Geometry check sheet. Reference: the model listing, model coordinates, mm. Face numbers are marked on the shaded views. A direction names the side the tool comes from. Coordinates: 2 decimals unless noted, no trailing zeros. Write each loop counter-clockwise with the first axis right and the second up, starting at its lowest first coordinate (ties: lowest second). Pieces come first, ordered by that corner, then holes. Notation, with made-up numbers: M 52.5,88 L 75.5,88 A23 ccw 75.5,114 Z; hole C 58.25,21.5 d10. An arc over 180 degrees is marked long. Write each question's results on one line, items separated by ' | '.
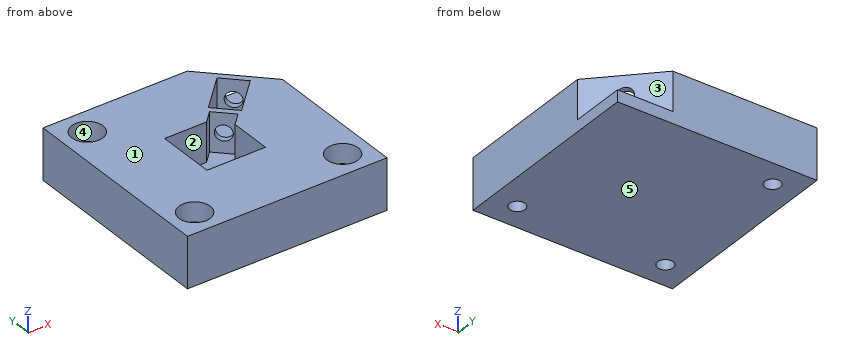
```python
from build123d import *

# Parameters (mm, degrees)
F0_W      = 51.2
F0_H      = 51.2
F0_R      = 2
F1_DEPTH  = 3
F2_R      = 2
F3_DEPTH  = 5
F4_R      = 4
F5_DEPTH  = 5
F6_R      = 2
F7_DEPTH  = 2
F8_R      = 3.5
F9_DEPTH  = 11
F10_R     = 2
F11_DEPTH = 4
F13_DEPTH = 9


with BuildPart() as f1:
    # F0 (on Top) → F1 (new body)
    with BuildSketch(Plane.XY):
        Rectangle(F0_W, F0_H)
        with Locations((-19, -19)):
            Circle(F0_R, mode=Mode.SUBTRACT)
        with Locations((19, -19)):
            Circle(F0_R, mode=Mode.SUBTRACT)
        with Locations((-19, 19)):
            Circle(F0_R, mode=Mode.SUBTRACT)
    extrude(amount=F1_DEPTH)

    # F2 (on face) → F3 (join)
    with BuildSketch(Plane.XY.offset(3)):
        Polygon((11.4, 25.6), (-25.6, 25.6), (-25.6, -25.6), (25.6, -25.6), (25.6, 11.4), align=None)
        with Locations((-19, -19)):
            Circle(F2_R, mode=Mode.SUBTRACT)
        with Locations((19, -19)):
            Circle(F2_R, mode=Mode.SUBTRACT)
        with Locations((-19, 19)):
            Circle(F2_R, mode=Mode.SUBTRACT)
        Polygon((-7.5, -7.5), (-7.5, 7.5), (3.2573593129, 7.5), (6.0857864376, 10.3284271247), (10.3284271247, 6.0857864376), (7.5, 3.2573593129), (7.5, -7.5), align=None, mode=Mode.SUBTRACT)
    extrude(amount=F3_DEPTH)

    # F4 (on face) → F5 (join)
    with BuildSketch(Plane.XY.offset(8)):
        Polygon((11.4, 25.6), (-25.6, 25.6), (-25.6, -25.6), (25.6, -25.6), (25.6, 11.4), align=None)
        with Locations((-19, -19)):
            Circle(F4_R, mode=Mode.SUBTRACT)
        with Locations((19, -19)):
            Circle(F4_R, mode=Mode.SUBTRACT)
        with Locations((-19, 19)):
            Circle(F4_R, mode=Mode.SUBTRACT)
        Polygon((-7.5, -7.5), (-7.5, 7.5), (3.2573593129, 7.5), (6.0857864376, 10.3284271247), (10.3284271247, 6.0857864376), (7.5, 3.2573593129), (7.5, -7.5), align=None, mode=Mode.SUBTRACT)
    extrude(amount=F5_DEPTH)

    # F6 (on face) → F7 (cut)
    with BuildSketch(Plane(origin=(18.5, 18.5, 0), x_dir=(-0.7071067812, 0.7071067812, 0), z_dir=(0.7071067812, 0.7071067812, 0))):
        with Locations((0, 8)):
            Circle(F6_R)
    extrude(amount=-F7_DEPTH, mode=Mode.SUBTRACT)

    # F8 (on face) → F9 (cut)
    with BuildSketch(Plane(origin=(17.0857864376, 17.0857864376, 0), x_dir=(-0.7071067812, 0.7071067812, 0), z_dir=(0.7071067812, 0.7071067812, 0))):
        with Locations((0, 8)):
            Circle(F8_R)
    extrude(amount=-F9_DEPTH, mode=Mode.SUBTRACT)

    # F10 (on face) → F11 (cut)
    with BuildSketch(Plane(origin=(8.2071067812, 8.2071067812, 0), x_dir=(0.7071067812, -0.7071067812, 0), z_dir=(-0.7071067812, -0.7071067812, 0))):
        with Locations((0, 8)):
            Circle(F10_R)
    extrude(amount=-F11_DEPTH, mode=Mode.SUBTRACT)

    # F12 (on face) → F13 (cut)
    with BuildSketch(Plane.XY.offset(13)):
        Polygon((14.9213203436, 19.8710678119), (6.7928932188, 11.7426406871), (11.7426406871, 6.7928932188), (19.8710678119, 14.9213203436), align=None)
    extrude(amount=-F13_DEPTH, mode=Mode.SUBTRACT)


solid = f1.part
```
Q1. Mould release check, pull along Y, two halves, no side actions. Record for the marked faces 1, 2 and 3: pulls with the +Y half, pulls with the -Y half, needs draft (parallel to the pull), parting line crosses it, or undercut.
Geometry check:
face 1: needs draft | face 2: undercut | face 3: pulls with the +Y half
Q2. Access from +Z, -Z, +X, -X, +Y, -Y to the whole of each face (thin tool, end or side, straight path). Record for the marked faces 4 and 5.
Geometry check:
face 4: +Z | face 5: -Z, +X, -X, +Y, -Y
Q3. Sectioned sample at C-C on x = 0. Record the cut outline in (y, z), and give its area (3 significant figures).
Geometry check:
outline: M -25.6,0 L 25.6,0 L 25.6,13 L 7.5,13 L 7.5,3 L -7.5,3 L -7.5,13 L -25.6,13 Z | area: 516 mm2
Q4. Scan lines: probe 1 along Y at (x, z) = (-19, 10.7); probe 2 along X at (y, z) = (2.5, 3.5); probe 3 along Y at (x, z) = (19, 5.25). Record each from-to range of solid material in increasing order.
Geometry check:
probe 1: y = -25.6 to -23, -15 to 15, 23 to 25.6 | probe 2: x = -25.6 to -7.5, 7.5 to 25.6 | probe 3: y = -25.6 to -21, -17 to 14.05, 15.79 to 18
Q5. Depth check by flat-ended pin: P1, Ø5, axis at x = -2, y = 4, coming from the +Z side; P2, Ø4, axis at x = 20, y = -20.5, coming from the +Z side. Enter the tip coordinate at first touch or a pass-through.
Geometry check:
P1: stops at z = 3 | P2: stops at z = 8
Q6. Sectioned sample at A-A on y = -19. Record the cut outline in (x, z), and give its area (3 significant figures).
Geometry check:
outline: M -25.6,0 L -21,0 L -21,8 L -23,8 L -23,13 L -25.6,13 Z; M -17,0 L 17,0 L 17,8 L 15,8 L 15,13 L -15,13 L -15,8 L -17,8 Z; M 21,0 L 25.6,0 L 25.6,13 L 23,13 L 23,8 L 21,8 Z | area: 522 mm2
